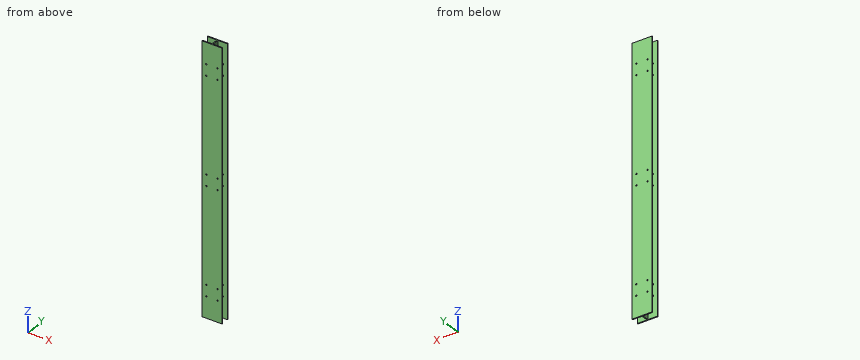
```python
from build123d import *

# Parameters (mm, degrees)
BOSS_EXTRUDE4_DEPTH       = 1200
CUT_EXTRUDE4_REACH        = 1203.096
SKETCH8_R                 = 3
LPATTERN1_COUNT           = 2
LPATTERN1_PITCH           = 480
LPATTERN1_COL_COUNT       = 2
LPATTERN1_COL_PITCH       = 480
SKETCH16_R                = 3
CUT_EXTRUDE11_DEPTH       = 1202.509467295
LPATTERN3_COUNT           = 2
LPATTERN3_PITCH           = 50
LPATTERN3_COUNT_DIR2      = 2
LPATTERN3_PITCH_DIR2      = 50
LPATTERN4_COUNT           = 3
LPATTERN4_PITCH           = 480
LPATTERN4_COPY_1_SKETCH_R = 3
LPATTERN4_COPY_1_DEPTH    = 1202.509467295
LPATTERN4_COPY_2_SKETCH_R = 3
LPATTERN4_COPY_2_DEPTH    = 1202.509467295
LPATTERN4_COPY_3_SKETCH_R = 3
LPATTERN4_COPY_3_DEPTH    = 1202.509467295
LPATTERN4_COPY_4_SKETCH_R = 3
LPATTERN4_COPY_4_DEPTH    = 1202.509467295
LPATTERN4_COPY_5_SKETCH_R = 3
LPATTERN4_COPY_5_DEPTH    = 1202.509467295
LPATTERN4_COPY_6_SKETCH_R = 3
LPATTERN4_COPY_6_DEPTH    = 1202.509467295
SKETCH25_R                = 2.1
CUT_EXTRUDE18_DEPTH       = 10


with BuildPart() as part:
    # Sketch1_6 → Boss-Extrude4 (new body)
    with BuildSketch(Plane.XY):
        Polygon((-2.25, 15.5), (-45, 15.5), (-45, 20), (45, 20), (45, 15.5), (2.25, 15.5), (2.25, -15.5), (45, -15.5), (45, -20), (-45, -20), (-45, -15.5), (-2.25, -15.5), align=None)
    extrude(amount=BOSS_EXTRUDE4_DEPTH)

    # Sketch8 → Cut-Extrude4 (cut, up to next)
    with BuildSketch(Plane(origin=(2.25, 0, 0), x_dir=(0, 0, -1), z_dir=(1, 0, 0)), mode=Mode.PRIVATE) as cut_extrude4_sk1:
        with Locations((-580.75, 0)):
            Circle(SKETCH8_R)
    cut_extrude4_tool1 = extrude(cut_extrude4_sk1.sketch, amount=-CUT_EXTRUDE4_REACH, mode=Mode.PRIVATE) & part.part
    cut_extrude4 = cut_extrude4_tool1.solids().sort_by_distance((2.25, 0, 580.75))[0]
    add(cut_extrude4, mode=Mode.SUBTRACT)

    # LPattern1: Cut-Extrude4 ×2
    with Locations(*[(0, 0, i * LPATTERN1_PITCH) for i in range(1, LPATTERN1_COUNT)]):
        add(cut_extrude4, mode=Mode.SUBTRACT)

    # LPattern1 col: Cut-Extrude4 ×2
    with Locations(*[(0, 0, -i * LPATTERN1_COL_PITCH) for i in range(1, LPATTERN1_COL_COUNT)]):
        add(cut_extrude4, mode=Mode.SUBTRACT)

    # Sketch16 → Cut-Extrude11 (cut, through all)
    with BuildSketch(Plane(origin=(0, 20, 0), x_dir=(1, 0, 0), z_dir=(0, 1, 0))):
        with Locations(Location((25, -95, 0), (0, 0, 270))):
            Circle(SKETCH16_R)
    cut_extrude11 = extrude(amount=-CUT_EXTRUDE11_DEPTH, mode=Mode.SUBTRACT)

    # LPattern3: Cut-Extrude11 2 × 2
    with Locations(*[(-j * LPATTERN3_PITCH_DIR2, 0, i * LPATTERN3_PITCH) for i in range(LPATTERN3_COUNT) for j in range(LPATTERN3_COUNT_DIR2) if (i, j) != (0, 0)]):
        add(cut_extrude11, mode=Mode.SUBTRACT)

    # LPattern4: Cut-Extrude11 ×3
    with Locations(*[(0, 0, i * LPATTERN4_PITCH) for i in range(1, LPATTERN4_COUNT)]):
        add(cut_extrude11, mode=Mode.SUBTRACT)

    # LPattern4 copy 1 sketch → LPattern4 copy 1 (cut, through all)
    with BuildSketch(Plane(origin=(-50, 20, 480), x_dir=(1, 0, 0), z_dir=(0, 1, 0))):
        with Locations(Location((25, -95, 0), (0, 0, 270))):
            Circle(LPATTERN4_COPY_1_SKETCH_R)
    extrude(amount=-LPATTERN4_COPY_1_DEPTH, mode=Mode.SUBTRACT)

    # LPattern4 copy 2 sketch → LPattern4 copy 2 (cut, through all)
    with BuildSketch(Plane(origin=(-50, 20, 960), x_dir=(1, 0, 0), z_dir=(0, 1, 0))):
        with Locations(Location((25, -95, 0), (0, 0, 270))):
            Circle(LPATTERN4_COPY_2_SKETCH_R)
    extrude(amount=-LPATTERN4_COPY_2_DEPTH, mode=Mode.SUBTRACT)

    # LPattern4 copy 3 sketch → LPattern4 copy 3 (cut, through all)
    with BuildSketch(Plane(origin=(0, 20, 530), x_dir=(1, 0, 0), z_dir=(0, 1, 0))):
        with Locations(Location((25, -95, 0), (0, 0, 270))):
            Circle(LPATTERN4_COPY_3_SKETCH_R)
    extrude(amount=-LPATTERN4_COPY_3_DEPTH, mode=Mode.SUBTRACT)

    # LPattern4 copy 4 sketch → LPattern4 copy 4 (cut, through all)
    with BuildSketch(Plane(origin=(0, 20, 1010), x_dir=(1, 0, 0), z_dir=(0, 1, 0))):
        with Locations(Location((25, -95, 0), (0, 0, 270))):
            Circle(LPATTERN4_COPY_4_SKETCH_R)
    extrude(amount=-LPATTERN4_COPY_4_DEPTH, mode=Mode.SUBTRACT)

    # LPattern4 copy 5 sketch → LPattern4 copy 5 (cut, through all)
    with BuildSketch(Plane(origin=(-50, 20, 530), x_dir=(1, 0, 0), z_dir=(0, 1, 0))):
        with Locations(Location((25, -95, 0), (0, 0, 270))):
            Circle(LPATTERN4_COPY_5_SKETCH_R)
    extrude(amount=-LPATTERN4_COPY_5_DEPTH, mode=Mode.SUBTRACT)

    # LPattern4 copy 6 sketch → LPattern4 copy 6 (cut, through all)
    with BuildSketch(Plane(origin=(-50, 20, 1010), x_dir=(1, 0, 0), z_dir=(0, 1, 0))):
        with Locations(Location((25, -95, 0), (0, 0, 270))):
            Circle(LPATTERN4_COPY_6_SKETCH_R)
    extrude(amount=-LPATTERN4_COPY_6_DEPTH, mode=Mode.SUBTRACT)

    # Sketch25 → Cut-Extrude18 (cut)
    with BuildSketch(Plane(origin=(2.25, 0, 0), x_dir=(0, 0, -1), z_dir=(1, 0, 0))):
        with Locations((-614.63, 0)):
            Circle(SKETCH25_R)
        with Locations((-632.63, 0)):
            Circle(SKETCH25_R)
    extrude(amount=-CUT_EXTRUDE18_DEPTH, mode=Mode.SUBTRACT)


solid = part.part
```
The listing builds one solid part. Answer for the finished solid, in the listing's coordinates (mm). Round coordinates to 2 decimals unless told otherwise and drop trailing zeros. Loops run counter-clockwise (first coordinate to the right, second up) from the corner with the lowest first, then second, coordinate; pieces in that order, holes last.
Q1. Section A-A, the plane z = 831 is taken. Determine the outline of the cut face in (x, y), then the cut area to 4 significant figures.
Q2. Find the intervals of material crossed by line 1 (X direction, y = 18.65, z = 575); line 2 (Y direction, x = 8, z = 51.5); line 3 (X direction, y = -8, z = 556), in increasing order.
Q3. Given pin 1 Ø12 at (x, y) = (-18, 6.5) entering from -Z; pin 2 Ø12 at (y, z) = (-6.5, 432) entering from +X; pin 3 Ø9.5 at (y, z) = (-6.5, 431) entering from -X, each flat-ended and moving along its own axis, determine where each tip first touches the part or whether it passes through.
Completed:
1. outline: (-45, -20) - (45, -20) - (45, -15.5) - (2.25, -15.5) - (2.25, 15.5) - (45, 15.5) - (45, 20) - (-45, 20) - (-45, 15.5) - (-2.25, 15.5) - (-2.25, -15.5) - (-45, -15.5) - close
1. area: 949.5 mm2
2. line 1: x = -45 to -28, -22 to 22, 28 to 45
2. line 2: y = -20 to -15.5, 15.5 to 20
2. line 3: x = -2.25 to 2.25
3. pin 1: passes through
3. pin 2: stops at x = 2.25
3. pin 3: stops at x = -2.25
